Can you work these out from the model? Positions are in its coordinate system, mm. A direction names the side the tool comes from. Give positions to 0.01 mm unless a question says otherwise; leave off trailing zeros. Answer as CSV lines item,"result".
```python
from build123d import *

# Parameters (mm, degrees)
F0_R     = 1.55
F0_R_2   = 11.8
F1_DEPTH = 1.27
F3_DEPTH = 0.254
F4_SIZE  = 1.26999


# Not quite as in the source:
# - a fillet or chamfer is up to 0.001 mm smaller than in the source, because OpenCascade refuses the exact size


with BuildPart() as f1:
    # F0 (on Front) → F1 (new body)
    with BuildSketch(Plane.XZ):
        with BuildLine():
            ThreePointArc((0, 3.175), (0.9299359697, 0.9299359697), (3.175, 0))
            Line((3.175, 0), (31.025, 0))
            ThreePointArc((31.025, 0), (33.2700640303, 0.9299359697), (34.2, 3.175))
            Line((34.2, 3.175), (34.2, 36.025))
            ThreePointArc((34.2, 36.025), (33.2700640303, 38.2700640303), (31.025, 39.2))
            Line((31.025, 39.2), (3.175, 39.2))
            ThreePointArc((3.175, 39.2), (0.9299359697, 38.2700640303), (0, 36.025))
            Line((0, 36.025), (0, 3.175))
        make_face()
        with Locations((26.5996, 7.5985)):
            Circle(F0_R, mode=Mode.SUBTRACT)
        with Locations((7.6004, 31.6015)):
            Circle(F0_R, mode=Mode.SUBTRACT)
        with Locations((17.1, 19.6)):
            Circle(F0_R_2, mode=Mode.SUBTRACT)
    extrude(amount=F1_DEPTH)

    # F2 (on face) → F3 (cut)
    with BuildSketch(Plane.XZ.offset(1.27)):
        with BuildLine():
            Line((27.025, 35.2), (7.175, 35.2))
            ThreePointArc((7.175, 35.2), (4.9299359697, 34.2700640303), (4, 32.025))
            Line((4, 32.025), (4, 7.175))
            ThreePointArc((4, 7.175), (4.9299359697, 4.9299359697), (7.175, 4))
            Line((7.175, 4), (27.025, 4))
            ThreePointArc((27.025, 4), (29.2700640303, 4.9299359697), (30.2, 7.175))
            Line((30.2, 7.175), (30.2, 32.025))
            ThreePointArc((30.2, 32.025), (29.2700640303, 34.2700640303), (27.025, 35.2))
        make_face()
    extrude(amount=-F3_DEPTH, mode=Mode.SUBTRACT)

    # F4 (size 1.27 in the source; OpenCascade refuses exactly that, so slightly less here)
    f4_edges = [f1.edges().sort_by_distance(p)[0] for p in [
        (34.2, -1.27, 19.6),
    ]]
    chamfer(f4_edges, length=F4_SIZE)


solid = f1.part
```
1) I'm going to push a flat-ended pin straight in: P1, Ø13, axis at x = 11.5, z = 19, coming from the -Y side. Where does the tip first touch, or does it pass through?
Answer block:
P1,"y = -1.02"
2) Which directions (+Z, -Z, +X, -X, +Y, -Y) give clear straight access to the entire face, cutting with the end or side of a thin tool? Please do faces 1 (the flat face through (9, 0, 29)), 2 (the flat face through (5, -1.016, 20)).
Answer block:
face 1,"+Z, -Z, +X, -X, +Y"
face 2,"-Y"
3) I want a section at C-C on y = -0.6. Count the separate pieces of the cut face and the enclosed holes in it, plus the area to 3 significant figures.
Answer block:
separate pieces,"1"
enclosed holes,"3"
area,"796 mm2"
4) If we mould it in two halves opening along Z, with no side actions, what happens to faces 3 (the conical face through (32.746, -0.767, 37.709)), 4 (the cylindrical face through (7.4, -0.5, 33.14)), 5 (the flat face through (17, -1, 1))? For each: +Z half, -Z half, draft (parallel to the pull), parting line (faces both ways), or undercut.
Answer block:
face 3,"+Z half"
face 4,"undercut"
face 5,"-Z half"
5) I need wall thicknesses on line 1 along Z through (x, y) = (7.5, -0.6); line 2 along Y through (x, z) = (18.5, 5); line 3 along Z through (x, y) = (12.5, -0.95). Which ranges of each line are inside material? Lowest first, please. Write a range as [from, to].
Answer block:
line 1,"[0.6, 12.74], [26.46, 30.05], [33.15, 38.6]"
line 2,"[-1.02, 0]"
line 3,"[0.95, 8.73], [30.47, 38.25]"
